```python
from build123d import *

# Parameters (mm, degrees)
F0_R     = 60
F1_DEPTH = 25


with BuildPart() as f1:
    # F0 (on Top) → F1 (new body)
    with BuildSketch(Plane.XY):
        Circle(F0_R)
        with BuildLine():
            ThreePointArc((-1.842674, -31.245442), (-4.150552, -27.526351), (-1.842674, -23.80726))
            Line((-1.842674, -23.80726), (-1.842674, -31.245442))
        make_face(mode=Mode.SUBTRACT)
        with BuildLine():
            ThreePointArc((-1.842674, -55.969675), (-56, 0), (-1.842674, 55.969675))
            Line((-1.842674, 55.969675), (-1.842674, -18.756511))
            ThreePointArc((-1.842674, -18.756511), (-8.961336, -27.526351), (-1.842674, -36.296191))
            Line((-1.842674, -36.296191), (-1.842674, -55.969675))
        make_face(mode=Mode.SUBTRACT)
        with BuildLine():
            Line((1.842674, -31.245442), (1.842674, -23.80726))
            ThreePointArc((1.842674, -23.80726), (4.150552, -27.526351), (1.842674, -31.245442))
        make_face(mode=Mode.SUBTRACT)
        with BuildLine():
            Line((1.842674, -18.756511), (1.842674, 55.969675))
            ThreePointArc((1.842674, 55.969675), (56, 0), (1.842674, -55.969675))
            Line((1.842674, -55.969675), (1.842674, -36.296191))
            ThreePointArc((1.842674, -36.296191), (8.961336, -27.526351), (1.842674, -18.756511))
        make_face(mode=Mode.SUBTRACT)
    extrude(amount=F1_DEPTH)


solid = f1.part
```
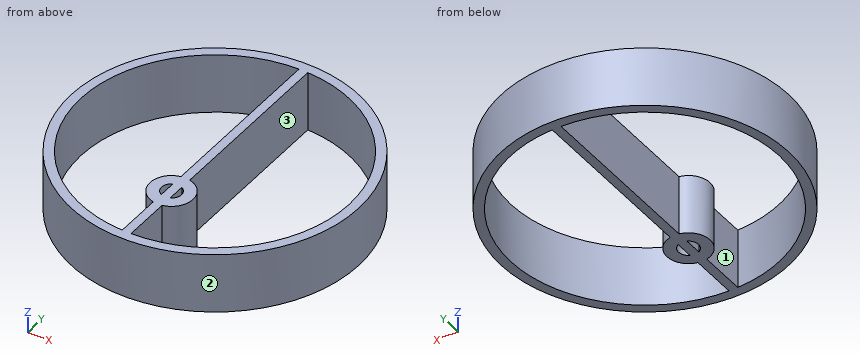
Check sheet for the modelled part. Datum: model origin and axes. Units: mm. Face numbers are marked on the shaded views. Give positions to 0.01 mm unless a question says otherwise; leave off trailing zeros. Loops run counter-clockwise (first coordinate to the right, second up) from the corner with the lowest first, then second, coordinate; pieces in that order, holes last. Notation, with made-up numbers: M -24.5,37 L 26.5,37 A29 cw 26.5,74 Z; hole C 70,-22.5 d2. An arc over 180 degrees is marked long. Answer in a Markdown table with one row per item.
1) Thickness scan on line 1 (Y direction, x = -6.5, z = 14); line 2 (X direction, y = 35, z = 11); line 3 (X direction, y = 21, z = 14). Record the ranges inside material, lowest first.
Solutions:
| item | result |
|---|---|
| line 1 | y = -59.65 to -55.62, -33.7 to -21.36, 55.62 to 59.65 |
| line 2 | x = -48.73 to -43.71, -1.84 to 1.84, 43.71 to 48.73 |
| line 3 | x = -56.2 to -51.91, -1.84 to 1.84, 51.91 to 56.2 |
2) Cross-section at D-D (x = -19.5). Enter the section's corners in (y, z).
Solutions:
| item | result |
|---|---|
| outline | M -56.74,0 L -52.5,0 L -52.5,25 L -56.74,25 Z; M 52.5,0 L 56.74,0 L 56.74,25 L 52.5,25 Z |
3) Cross-section at B-B (x = 14). Enter the section's corners in (y, z).
Solutions:
| item | result |
|---|---|
| outline | M -58.34,0 L -54.22,0 L -54.22,25 L -58.34,25 Z; M 54.22,0 L 58.34,0 L 58.34,25 L 54.22,25 Z |
4) Mould release check, pull along X, two halves, no side actions. Record for the marked faces 1, 2 and 3: released by +X, released by -X, zero draft, split by the parting line, or undercut.
Solutions:
| item | result |
|---|---|
| face 1 | undercut |
| face 2 | split by the parting line |
| face 3 | undercut |
5) Cross-section at A-A (y = 0). Enter the section's corners in (x, z).
Solutions:
| item | result |
|---|---|
| outline | M -60,0 L -56,0 L -56,25 L -60,25 Z; M -1.84,0 L 1.84,0 L 1.84,25 L -1.84,25 Z; M 56,0 L 60,0 L 60,25 L 56,25 Z |
6) Depth check by flat-ended pin: pin 1 (1.5 mm diameter, centred on x = -1, z = 6, fed in from -Y); pin 2 (3 mm diameter, centred on y = 12, z = 13, fed in from -X); pin 3 (10 mm diameter, centred on y = -47.5, z = 10.5, fed in from -X). Enter the tip coordinate at first touch or a pass-through.
Solutions:
| item | result |
|---|---|
| pin 1 | stops at y = -60 |
| pin 2 | stops at x = -59.07 |
| pin 3 | stops at x = -42.35 |
7) Cross-section at C-C (z = 21.75). Enter the section's corners in (x, y).
Solutions:
| item | result |
|---|---|
| outline | C 0,0 d120; hole M -1.84,-55.97 L -1.84,-36.3 A8.96 cw -1.84,-18.76 L -1.84,55.97 A56 ccw Z; hole M -1.84,-31.25 L -1.84,-23.81 A4.15 ccw Z; hole M 1.84,-55.97 A56 ccw 1.84,55.97 L 1.84,-18.76 A8.96 cw 1.84,-36.3 Z; hole M 1.84,-31.25 A4.15 ccw 1.84,-23.81 Z |
